Autodesk Inventor part; units mm, degrees
ref_plane "Work Plane1" through (5.08, 40.767, 0) normal (1, 0, 0) x (0, 0, -1)
ref_plane "YZ Plane" through (0, 0, 0) normal (1, 0, 0) x (0, 1, 0)
ref_plane "XZ Plane" through (0, 0, 0) normal (0, 1, 0) x (-1, 0, 0)
sketch "Sketch1" plane through (0, 0, 0) normal (0, 0, 1) x (1, 0, 0)
  line L0 (-38.227, 38.227) -> (38.227, 38.227)
  line L1 (38.227, 38.227) -> (38.227, -38.227)
  line L2 (38.227, -38.227) -> (-38.227, -38.227)
  line L3 (-38.227, -38.227) -> (-38.227, 38.227)
  point P0 (0, 0)
  dimension "d0" = 76.454
  dimension "d1" = 76.454
  dimension "d2" = 38.227
  dimension "d3" = 38.227
extrude "Extrusion1" add sketch "Sketch1" along normal blind 2.54
sketch "Sketch2" plane through (0, 0, 2.54) normal (0, 0, 1) x (1, 0, 0)
  line L0 (-38.227, -38.227) -> (38.227, -38.227)
  line L1 (38.227, -38.227) -> (38.227, 38.227)
  line L2 (38.227, 38.227) -> (-38.227, 38.227)
  line L3 (-38.227, 38.227) -> (-38.227, -38.227)
  line L4 (-40.767, 40.767) -> (40.767, 40.767)
  line L5 (40.767, 40.767) -> (40.767, -40.767)
  line L6 (40.767, -40.767) -> (-40.767, -40.767)
  line L7 (-40.767, -40.767) -> (-40.767, 40.767)
  point P0 (0, 0)
  dimension "d6" = 2.54
extrude "Extrusion2" add sketch "Sketch2" against normal blind 25.4
sketch "Sketch3" plane through (-40.767, 40.767, 2.54) normal (0, 1, 0) x (1, 0, 0)
  line L0 (81.534, 0) -> (0, 0)
  line L1 (81.534, 0) -> (81.534, 25.4)
  line L2 (0, 25.4) -> (81.534, 25.4)
  line L3 (0, 0) -> (0, 25.4)
  line L4 (78.994, 2.54) -> (2.54, 2.54)
  line L5 (2.54, 2.54) -> (2.54, 25.4)
  line L6 (78.994, 2.54) -> (78.994, 25.4)
  line L7 (33.147, 2.54) -> (32.639, 2.54)
  line L8 (32.639, 2.54) -> (32.639, 25.4)
  line L9 (32.639, 25.4) -> (33.147, 25.4)
  line L10 (33.147, 25.4) -> (33.147, 2.54)
  line L11 (78.994, 25.4) -> (2.54, 25.4)
  line L12 (48.387, 2.54) -> (48.895, 2.54)
  line L13 (48.895, 2.54) -> (48.895, 25.4)
  line L14 (48.895, 25.4) -> (48.387, 25.4)
  line L15 (48.387, 25.4) -> (48.387, 2.54)
  point P0 (40.767, 2.54)
  point P1 (40.767, 2.54)
  dimension "d9" = 15.24
  dimension "d10" = 7.62
  dimension "d11" = 0.508
  dimension "d12" = 0.508
extrude "Extrusion3" cut sketch "Sketch3" against normal blind 25.4 contours L13 L4 L15 L2 | L2 L10 L4 L8
ref_plane "Work Plane1" through (5.08, 40.767, 0) normal (1, 0, 0) x (0, 0, -1)
sketch "Sketch6" plane through (5.08, 40.767, 0) normal (1, 0, 0) x (0, 0, -1)
  line L0 (0, -2.54) -> (22.86, -2.54)
  line L1 (0, 0) -> (0, -2.54)
  line L2 (22.86, 0) -> (0, 0)
  line L3 (22.86, -2.54) -> (22.86, 0)
  line L4 (-2.54, 0) -> (-2.54, -81.534)
  line L5 (-2.54, 0) -> (22.86, 0)
  line L6 (22.86, -81.534) -> (22.86, 0)
  line L7 (-2.54, -81.534) -> (22.86, -81.534)
  line L8 (0, -2.54) -> (0, -78.994)
  line L9 (0, -78.994) -> (22.86, -78.994)
  line L10 (22.86, -2.54) -> (22.86, -78.994)
  line L11 (0, -2.54) -> (22.86, -2.54)
  line L12 (3.2004, -2.54) -> (3.2004, -3.81)
  line L13 (3.2004, -3.81) -> (6.35, -2.54)
  point P0 (0, -40.767)
  point P1 (6.35, -2.54)
  point P2 (3.2004, -2.54)
  dimension "d20" = 3.2004
  dimension "d21" = 3.1496
  dimension "d22" = 1.27
extrude "Extrusion4" add sketch "Sketch6" against normal blind 10.16 contours L0 L13 L12
sketch "Sketch7" plane through (7.62, 40.767, 0) normal (1, 0, 0) x (0, 0, -1)
  line L0 (0, -2.54) -> (22.86, -2.54)
  line L1 (0, 0) -> (0, -2.54)
  line L2 (22.86, 0) -> (0, 0)
  line L3 (22.86, -2.54) -> (22.86, 0)
  line L4 (22.86, 5.5075) -> (16.1237, 0)
  line L5 (-2.54, 0) -> (22.86, 0)
  line L6 (18.6021, 0) -> (22.86, 3.4812)
  line L7 (22.86, 3.4812) -> (22.86, 5.5075)
  point P0 (0, -40.767)
extrude "Extrusion5" add sketch "Sketch7" against normal blind 15.24 contours L4 L7 L6 L2
equation "\"d12\" = d11"
properties part number "Part_6_lid"
The listing builds one solid part. Answer for the finished solid, in the listing's coordinates (mm). A direction names the side the tool comes from. Give positions to 0.01 mm unless a question says otherwise; leave off trailing zeros. Order: outer loops, then holes, each group sorted by start corner. A loop starts at its lowest first (then second) coordinate and runs counter-clockwise, first axis right, second up.
Item 1: The part is cut by section B-B, the plane y = 24.5. Give the vertices of the cut face in (x, z).
From the geometry:
outline: (-40.77, -22.86) - (-38.23, -22.86) - (-38.23, 0) - (38.23, 0) - (38.23, -22.86) - (40.77, -22.86) - (40.77, 2.54) - (-40.77, 2.54) - close
Item 2: Find the intervals of material crossed by probe 1 along X at (y, z) = (6.5, -10.5); probe 2 along Z at (x, y) = (19, 15), in increasing order.
From the geometry:
probe 1: x = -40.77 to -38.23, 38.23 to 40.77
probe 2: z = 0 to 2.54
Item 3: Given pin 1 Ø7 at (x, z) = (0, -13) entering from +Y; pin 2 Ø7.5 at (x, z) = (8, -5) entering from +Y; pin 3 Ø4.5 at (x, z) = (3, -20) entering from +Y, each flat-ended and moving along its own axis, determine where each tip first touches the part or whether it passes through.
From the geometry:
pin 1: stops at y = 41.07
pin 2: stops at y = 40.77
pin 3: stops at y = 45.78
Item 4: For a pull along X with two mould halves and no side action, classify faces 1 (the face through (-1, 2, 0)), 2 (the face through (40.767, 1, -10)), 3 (the face through (-1, 40.767, -10)) as pulls with the +X half, pulls with the -X half, needs draft (parallel to the pull), parting line crosses it, or undercut.
From the geometry:
face 1: undercut
face 2: pulls with the +X half
face 3: needs draft
Item 5: The part is cut by section A-A, the plane z = -11. Give the vertices of the cut face in (x, y).
From the geometry:
outline: (-40.77, -40.77) - (40.77, -40.77) - (40.77, 40.77) - (8.13, 40.77) - (8.13, 38.23) - (38.23, 38.23) - (38.23, -38.23) - (-38.23, -38.23) - (-38.23, 38.23) - (-8.13, 38.23) - (-8.13, 40.77) - (-40.77, 40.77) - close; (-7.62, 38.23) - (7.62, 38.23) - (7.62, 40.77) - (-7.62, 40.77) - close
Item 6: Which of the six approach directions +Z, -Z, +X, -X, +Y, -Y give full straight-line access (tool end or side, diameter ignored) to faces 4 (the face through (-23, 38.227, -11)), 5 (the face through (7.62, 40.5, -14.1)), 6 (the face through (0, 40, -22.86))?
From the geometry:
face 4: -Z
face 5: -Z, +Y
face 6: -Z, +X, -X, +Y, -Y
